Geometry: see drawing. Coordinates: mm, zero at the bounding-box minimum. A direction names the side the tool comes from. Give positions to 0.01 mm unless a question says otherwise; leave off trailing zeros. Loops run counter-clockwise (first coordinate to the right, second up) from the corner with the lowest first, then second, coordinate; pieces in that order, holes last. Notation, with made-up numbers: M 44,34 L 89,34 A11 cw 89,43 Z; hole C 47,60 d9. An arc over 180 degrees is marked long. Put each result on its own line as item: value.
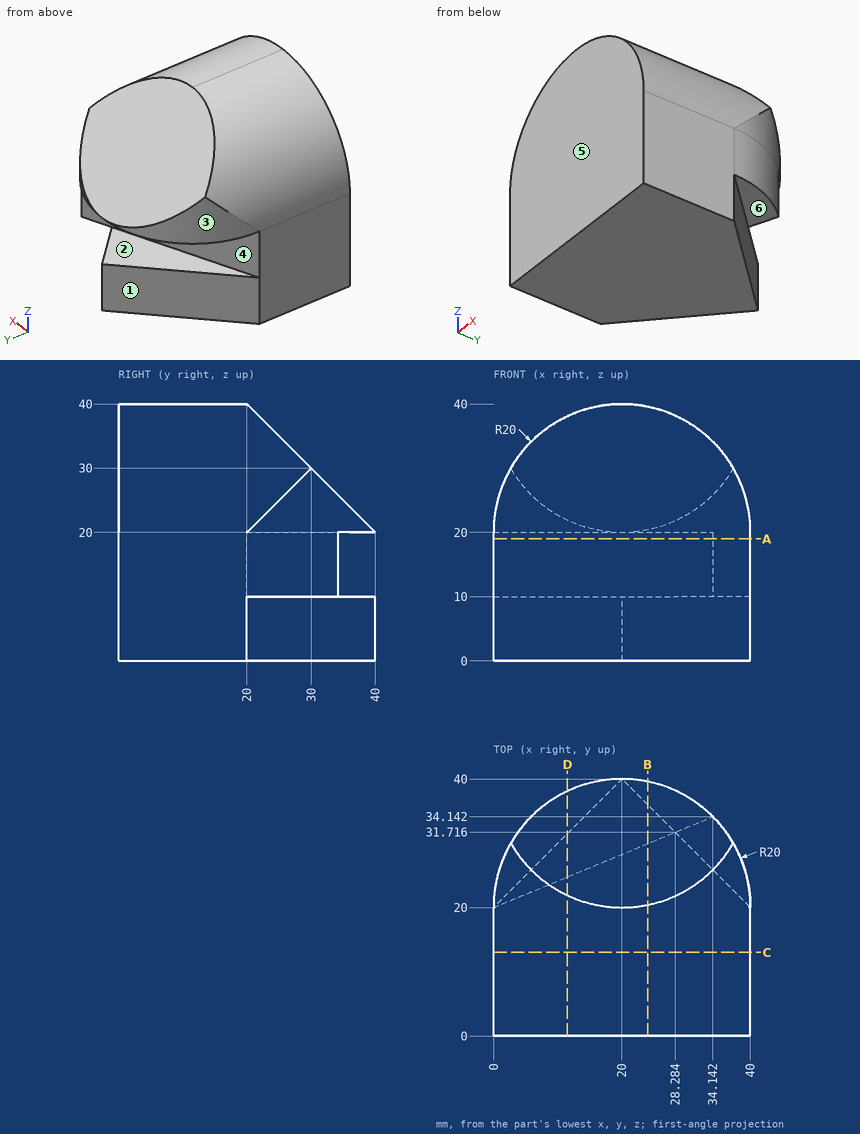
1. Section query C-C (y = 13). Output: boundary loops of the cut face in (x, z), plus the area to 3 significant figures.
Found:
outline: M 0,0 L 40,0 L 40,20 A20 ccw 20,40 A20 ccw 0,20 Z
area: 1,430 mm^2
2. Access query for the marked faces 1, 2 and 3. Directions: +Z, -Z, +X, -X, +Y, -Y. A direction counts if a zero-diameter tool reaches every point of the face in a straight line with its end or side. Return the directions, or none.
Found:
face 1: -Z, -X, +Y
face 2: -X, +Y
face 3: +Z, -Z, -X, +Y
3. Contact query for flat-ended pins moving along their axis: P1, Ø12, axis at x = 9.5, y = 24.5, coming from the -Z side; P2, Ø6, axis at x = 22.5, z = 22, coming from the +Y side; P3, Ø1.5, axis at x = 32, y = 5.5, coming from the +Z side; P4, Ø16, axis at x = 20, y = 31, coming from the +Z side. Output: stop coordinate, or through.
Found:
P1: z = 0
P2: y = 40
P3: z = 36.54
P4: z = 37
4. Section query B-B (x = 24). Output: boundary loops of the cut face in (y, z), plus the area to 3 significant figures.
Found:
outline: M 0,0 L 36,0 L 36,10 L 29.94,10 L 29.94,20 L 39.6,20 L 39.6,20.4 L 20.4,39.6 L 0,39.6 Z
area: 1,250 mm^2
5. Material intervals for line 1 (Z direction, x = 12, y = 19); line 2 (X direction, y = 26.5, z = 19) (1 decimal); line 3 (Z direction, x = 6.5, y = 12) (1 decimal), sorted ascending. Write a range as from..to.
Found:
line 1: 0..38.33
line 2: 15.7..38.9
line 3: 0..34.8
6. Section query D-D (x = 11.5). Output: boundary loops of the cut face in (y, z), plus the area to 3 significant figures.
Found:
outline: M 0,0 L 31.5,0 L 31.5,10 L 24.76,10 L 24.76,20 L 38.1,20 L 38.1,21.9 L 21.9,38.1 L 0,38.1 Z
area: 1,120 mm^2
7. Draft query along Z for the marked faces 4, 5 and 6. Return one class per face: pulls with the +Z half, pulls with the -Z half, needs draft (parallel to the pull), parting line crosses it, or undercut.
Found:
face 4: undercut
face 5: needs draft
face 6: pulls with the -Z half
8. Section query A-A (z = 19). Output: boundary loops of the cut face in (x, y).
Found:
outline: M 0,0 L 40,0 L 40,20 A20 ccw 34.14,34.14 L 0,20 Z
